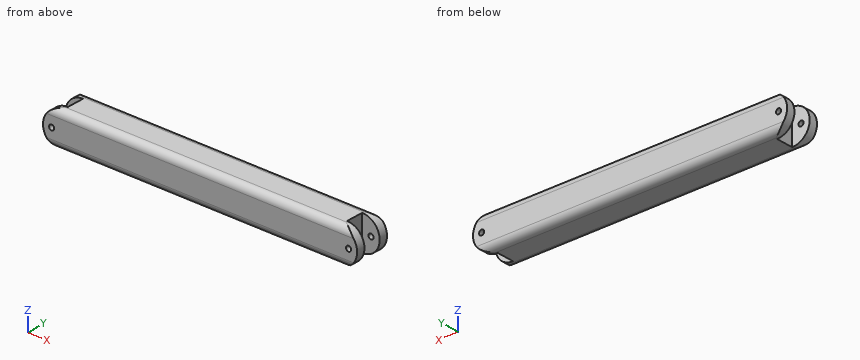
```python
from build123d import *

# Parameters (mm, degrees)
BOSS_EXTRUDE1_DEPTH = 228.4
SKETCH2_W           = 25.4
SKETCH2_H           = 25.4
CUT_EXTRUDE1_DEPTH  = 25
SKETCH4_R           = 3.75
CUT_EXTRUDE6_DEPTH  = 25


with BuildPart() as part:
    # Sketch1 → Boss-Extrude1 (new, symmetric)
    with BuildSketch(Plane(origin=(0, 0, 0), x_dir=(0, 0, -1), z_dir=(1, 0, 0))):
        with BuildLine():
            Line((-15, 25), (15, 25))
            ThreePointArc((15, 25), (22.071067812, 22.071067812), (25, 15))
            Line((25, 15), (25, -15))
            ThreePointArc((25, -15), (22.071067812, -22.071067812), (15, -25))
            Line((15, -25), (-15, -25))
            ThreePointArc((-15, -25), (-22.071067812, -22.071067812), (-25, -15))
            Line((-25, -15), (-25, 15))
            ThreePointArc((-25, 15), (-22.071067812, 22.071067812), (-15, 25))
        make_face()
    extrude(amount=BOSS_EXTRUDE1_DEPTH, both=True)

    # Sketch2 → Cut-Extrude1 (cut, symmetric)
    with BuildSketch(Plane.XY):
        with Locations((215.7, 0)):
            Rectangle(SKETCH2_W, SKETCH2_H)
        with Locations((-215.7, 0)):
            Rectangle(SKETCH2_W, SKETCH2_H)
    extrude(amount=CUT_EXTRUDE1_DEPTH, both=True, mode=Mode.SUBTRACT)

    # Sketch4 → Cut-Extrude6 (cut, symmetric)
    with BuildSketch(Plane(origin=(0, 0, 0), x_dir=(1, 0, 0), z_dir=(0, 1, 0))):
        with Locations(Location((-215.9, 0, 0), (0, 0, 270))):
            Circle(SKETCH4_R)
        with Locations(Location((215.9, 0, 0), (0, 0, 270))):
            Circle(SKETCH4_R)
        with BuildLine():
            Line((-203.4, 25), (-203.4, 45))
            ThreePointArc((-203.4, 45), (-248.4, 0), (-203.4, -45))
            Line((-203.4, -45), (-203.4, -25))
            ThreePointArc((-203.4, -25), (-228.4, 0), (-203.4, 25))
        make_face()
        with BuildLine():
            Line((203.4, 45), (203.4, 25))
            ThreePointArc((203.4, 25), (228.4, 0), (203.4, -25))
            Line((203.4, -25), (203.4, -45))
            ThreePointArc((203.4, -45), (248.4, 0), (203.4, 45))
        make_face()
    extrude(amount=CUT_EXTRUDE6_DEPTH, both=True, mode=Mode.SUBTRACT)


solid = part.part
```
Source: CAD feature listing. Evaluate the final solid. Frame: model axes, mm. Coordinates: 2 decimals unless noted, no trailing zeros. Loops run counter-clockwise (first coordinate to the right, second up) from the corner with the lowest first, then second, coordinate; pieces in that order, holes last. Notation, with made-up numbers: M -22.75,72 L 9.25,72 A16 ccw 9.25,89 Z; hole C -9,75.25 d10. An arc over 180 degrees is marked long. Put each result on its own line as item: value. Start each with the question number.
1) Cut plane C-C on y = -21. Return the cut outline in (x, z).
2) Cut plane B-B on x = -109. Return the cut outline in (y, z).
3) Cut plane A-A on x = 215.9. Return the cut outline in (y, z).
4) Ray query, L1, parallel to X at y = 19.25, z = 0; L2, parallel to X at y = -10.5, z = -6; L3, parallel to Z at x = -114.5, y = 15.5. Return the intervals inside material, ascending. Write a range as from..to.
5) Contact query for flat-ended pins moving along their axis: pin 1 Ø7.5 at (y, z) = (2, 12) entering from +X; pin 2 Ø20.5 at (y, z) = (1.5, 12) entering from -X. Output: stop coordinate, or through.
6) Cut plane D-D on z = -21. Return the cut outline in (x, y).
The answers:
1. outline: M -213.2,-23 L 213.2,-23 A25 ccw 213.2,23 L -213.2,23 A25 ccw Z; hole C -215.9,0 d7.5; hole C 215.9,0 d7.5
2. outline: M -25,-15 A10 ccw -15,-25 L 15,-25 A10 ccw 25,-15 L 25,15 A10 ccw 15,25 L -15,25 A10 ccw -25,15 Z
3. outline: M -25,-15 A10 ccw -22.47,-21.65 L -12.7,-21.65 L -12.7,-3.75 L -25,-3.75 Z; M -25,3.75 L -12.7,3.75 L -12.7,21.65 L -22.47,21.65 A10 ccw -25,15 Z; M 12.7,-21.65 L 22.47,-21.65 A10 ccw 25,-15 L 25,-3.75 L 12.7,-3.75 Z; M 12.7,3.75 L 25,3.75 L 25,15 A10 ccw 22.47,21.65 L 12.7,21.65 Z
4. L1: x = -228.4..-219.65, -212.15..212.15, 219.65..228.4
4. L2: x = -203..203
4. L3: z = -24.99..24.99
5. pin 1: stops at x = 203
5. pin 2: stops at x = -203
6. outline: M -216.96,-23 L 216.96,-23 L 216.96,-12.7 L 203,-12.7 L 203,12.7 L 216.96,12.7 L 216.96,23 L -216.96,23 L -216.96,12.7 L -203,12.7 L -203,-12.7 L -216.96,-12.7 Z
